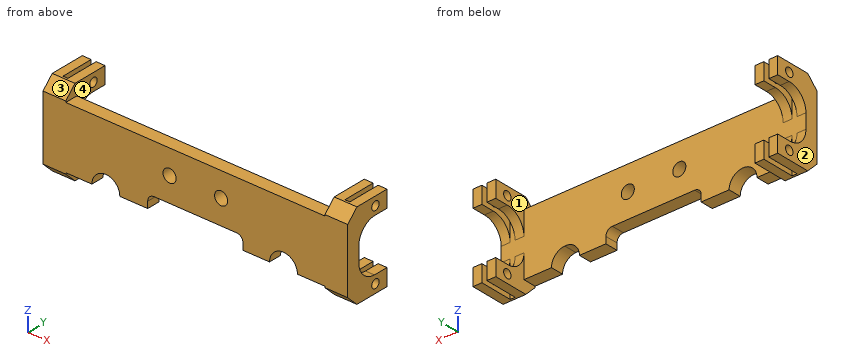
from build123d import *

# Parameters (mm, degrees)
BOSS_EXTRUDE1_DEPTH      = 3
SKETCH2_W                = 14.396583112
SKETCH2_H                = 3
BOSS_EXTRUDE2_DEPTH      = 8.6
SKETCH3_R                = 1
BOSS_EXTRUDE3_DEPTH      = 5.3
SKETCH4_W                = 1.15
SKETCH4_H                = 7.632118098
CUT_EXTRUDE1_DEPTH       = 26.3
CHAMFER1_SIZE            = 2.5
CUT_EXTRUDE2_DEPTH       = 10
CHAMFER1_OF_MIRROR1_SIZE = 2.5
CUT_EXTRUDE5_START       = -10
CUT_EXTRUDE5_DEPTH       = 10
BOSS_EXTRUDE4_DEPTH      = 3
SKETCH7_R                = 1.525
CUT_EXTRUDE6_DEPTH       = 41.163420863


with BuildPart() as part:
    # Sketch1 → Boss-Extrude1 (new body)
    with BuildSketch(Plane(origin=(0, 0, 0), x_dir=(1, 0, 0), z_dir=(0, 1, 0))):
        with BuildLine():
            Line((-26.88337521, 0), (-26.88337521, 14.396583112))
            Line((-26.88337521, 14.396583112), (-24.09337521, 14.396583112))
            ThreePointArc((-24.09337521, 14.396583112), (-20.84337521, 11.146583112), (-17.59337521, 14.396583112))
            Line((-17.59337521, 14.396583112), (0, 14.396583112))
            Line((0, 14.396583112), (0, 0))
            Line((0, 0), (-26.88337521, 0))
        make_face()
    boss_extrude1 = extrude(amount=BOSS_EXTRUDE1_DEPTH)

    # Sketch2 → Boss-Extrude2 (add)
    with BuildSketch(Plane.ZY.offset(26.88337521)):
        with Locations((-7.198291556, 1.5)):
            Rectangle(SKETCH2_W, SKETCH2_H)
    boss_extrude2 = extrude(amount=BOSS_EXTRUDE2_DEPTH)

    # Sketch3 → Boss-Extrude3 (add)
    with BuildSketch(Plane.ZY.offset(35.48337521)):
        with BuildLine():
            Line((1.532781983, 10.632118098), (-1.123291556, 10.632118098))
            Line((-1.123291556, 10.632118098), (-1.123291556, 10.557118098))
            Line((-1.123291556, 10.557118098), (-1.123291556, 7.547815402))
            ThreePointArc((-1.123291556, 7.547815402), (-2.349871735, 4.342215517), (-5.508799885, 3))
            Line((-5.508799885, 3), (-8.887750376, 3))
            ThreePointArc((-8.887750376, 3), (-11.934395079, 4.229921298), (-13.273291556, 7.230272374))
            Line((-13.273291556, 7.230272374), (-13.273291556, 10.557118098))
            Line((-13.273291556, 10.557118098), (-13.273291556, 10.632118098))
            Line((-13.273291556, 10.632118098), (-15.929365096, 10.632118098))
            Line((-15.929365096, 10.632118098), (-17.198291556, 10.632118098))
            Line((-17.198291556, 10.632118098), (-17.198291556, 7.5))
            Line((-17.198291556, 7.5), (-17.198291556, 0))
            Line((-17.198291556, 0), (-14.396583112, 0))
            Line((-14.396583112, 0), (0, 0))
            Line((0, 0), (2.801708444, 0))
            Line((2.801708444, 0), (2.801708444, 7.5))
            Line((2.801708444, 7.5), (2.801708444, 10.632118098))
            Line((2.801708444, 10.632118098), (1.532781983, 10.632118098))
        make_face()
        with Locations((-15.198291556, 7.5)):
            Circle(SKETCH3_R, mode=Mode.SUBTRACT)
        with Locations((0.801708444, 7.5)):
            Circle(SKETCH3_R, mode=Mode.SUBTRACT)
    boss_extrude3 = extrude(amount=-BOSS_EXTRUDE3_DEPTH)

    # Sketch4 → Cut-Extrude1 (cut)
    with BuildSketch(Plane.XY.offset(2.801708444)):
        with Locations((-32.83337521, 6.816059049)):
            Rectangle(SKETCH4_W, SKETCH4_H)
    cut_extrude1 = extrude(amount=-CUT_EXTRUDE1_DEPTH, mode=Mode.SUBTRACT)

    # Chamfer1
    chamfer1_edges = [part.edges().sort_by_distance(p)[0] for p in [
        (-32.83337521, 0, -17.198291556),
        (-32.83337521, 0, 2.801708444),
    ]]
    chamfer(chamfer1_edges, length=CHAMFER1_SIZE)

    # Sketch5 → Cut-Extrude2 (cut)
    with BuildSketch(Plane(origin=(0, 3, 0), x_dir=(1, 0, 0), z_dir=(0, 1, 0))):
        with BuildLine():
            Line((0, 11.381166784), (-9.598972409, 11.381166784))
            ThreePointArc((-9.598972409, 11.381166784), (-10.65963258, 11.820506612), (-11.098972409, 12.881166784))
            Line((-11.098972409, 12.881166784), (-11.098972409, 14.396583112))
            Line((-11.098972409, 14.396583112), (0, 14.396583112))
            Line((0, 14.396583112), (0, 11.381166784))
        make_face()
    cut_extrude2 = extrude(amount=-CUT_EXTRUDE2_DEPTH, mode=Mode.SUBTRACT)

    # Mirror1: Boss-Extrude1, Boss-Extrude2, Boss-Extrude3, Cut-Extrude1, Cut-Extrude2 across plane
    add(boss_extrude1.mirror(Plane(origin=(0, 0, 0), x_dir=(0, 0, 1), z_dir=(1, 0, 0))))
    add(boss_extrude2.mirror(Plane(origin=(0, 0, 0), x_dir=(0, 0, 1), z_dir=(1, 0, 0))))
    add(boss_extrude3.mirror(Plane(origin=(0, 0, 0), x_dir=(0, 0, 1), z_dir=(1, 0, 0))))
    add(cut_extrude1.mirror(Plane(origin=(0, 0, 0), x_dir=(0, 0, 1), z_dir=(1, 0, 0))), mode=Mode.SUBTRACT)
    add(cut_extrude2.mirror(Plane(origin=(0, 0, 0), x_dir=(0, 0, 1), z_dir=(1, 0, 0))), mode=Mode.SUBTRACT)

    # Chamfer1 of Mirror1
    chamfer1_of_mirror1_edges = [part.edges().sort_by_distance(p)[0] for p in [
        (32.83337521, 0, -17.198291556),
        (32.83337521, 0, 2.801708444),
    ]]
    chamfer(chamfer1_of_mirror1_edges, length=CHAMFER1_OF_MIRROR1_SIZE)

    # Sketch6 → Cut-Extrude5 (cut)
    with BuildSketch(Plane(origin=(0, 3, 0), x_dir=(1, 0, 0), z_dir=(0, 1, 0)).offset(CUT_EXTRUDE5_START)):
        with BuildLine():
            ThreePointArc((20.68337521, 11.150523963), (22.877361191, 12.155768528), (23.77337521, 14.396583112))
            ThreePointArc((23.77337521, 14.396583112), (20.52337521, 17.646583112), (17.27337521, 14.396583112))
            Line((17.27337521, 14.396583112), (17.59337521, 14.396583112))
            ThreePointArc((17.59337521, 14.396583112), (18.489389228, 12.155768528), (20.68337521, 11.150523963))
        make_face()
        with BuildLine():
            Line((17.59337521, 14.396583112), (17.27337521, 14.396583112))
            ThreePointArc((17.27337521, 14.396583112), (18.282560626, 12.042597131), (20.68337521, 11.150523963))
            ThreePointArc((20.68337521, 11.150523963), (18.489389228, 12.155768528), (17.59337521, 14.396583112))
        make_face()
    extrude(amount=CUT_EXTRUDE5_DEPTH, mode=Mode.SUBTRACT)

    # Sketch6<3> → Boss-Extrude4 (add, through all)
    with BuildSketch(Plane(origin=(0, 3, 0), x_dir=(1, 0, 0), z_dir=(0, 1, 0))):
        with BuildLine():
            Line((24.09337521, 14.396583112), (23.77337521, 14.396583112))
            ThreePointArc((23.77337521, 14.396583112), (22.877361191, 12.155768528), (20.68337521, 11.150523963))
            ThreePointArc((20.68337521, 11.150523963), (20.763350947, 11.147568474), (20.84337521, 11.146583112))
            ThreePointArc((20.84337521, 11.146583112), (23.141472249, 12.098486073), (24.09337521, 14.396583112))
        make_face()
    extrude(amount=-BOSS_EXTRUDE4_DEPTH)

    # Sketch7 → Cut-Extrude6 (cut, through all)
    with BuildSketch(Plane(origin=(0, 3, 0), x_dir=(1, 0, 0), z_dir=(0, 1, 0))):
        with Locations(Location((-6, 5.690583392, 0), (0, 0, 270))):
            Circle(SKETCH7_R)
        with Locations(Location((6, 5.690583392, 0), (0, 0, 90))):
            Circle(SKETCH7_R)
    extrude(amount=-CUT_EXTRUDE6_DEPTH, mode=Mode.SUBTRACT)


solid = part.part
CAD build for the part. Positions are in the model's coordinates, mm. Face numbers are marked on the shaded views. Coordinates: 2 decimals unless noted, no trailing zeros. Loops run counter-clockwise (first coordinate to the right, second up) from the corner with the lowest first, then second, coordinate; pieces in that order, holes last. Notation, with made-up numbers: (-26, 4) - (-14, 4) arc R27 ccw to (-14, 20) - close; hole circle Ø5 at (-10, 73). An arc over 180 degrees is marked (long way). Write item = value, one per line. Start each with the question number.
Q1. Drill centre lines: L1, parallel to X at y = 4.25, z = -16.5; L2, parallel to Z at x = 34.8, y = 7.5; L3, parallel to Z at x = 6, y = 2.45. Where is each one in solid material? Low to high.
Q2. Cut at C-C, the plane z = -12. List the corners of the cut face in (x, y), then the cut area to 3 significant figures.
Q3. Cut at D-D, the plane x = -25. List the corners of the cut face in (y, z).
Q4. Pull direction X, two halves, no side cores. Call the marked faces 1, 2, 3 and 4: pulls with the +X half, pulls with the -X half, needs draft (parallel to the pull), parting line crosses it, or undercut.
Q5. Cut at A-A, the plane y = 9.5. Give the number of separate pieces and of enclosed holes in the cut face, then the cut area to 3 significant figures.
Q6. Cut at B-B, the plane x = 6. List the corners of the cut face in (y, z), then the cut area to 3 significant figures.
Q7. Flat gauge pins, fed straight in: pin 1 Ø3 at (x, z) = (-4, -3) entering from -Y; pin 2 Ø1.2 at (y, z) = (7.5, 0.8) entering from -X; pin 3 Ø2.5 at (x, y) = (-12.5, 2) entering from -Z. Where does each tip first touch, or does it go through?
Computed:
q1.L1 = -35.48 to -33.41, -32.26 to -30.18, 30.18 to 32.26, 33.41 to 35.48
q1.L2 = -17.2 to -16.2, -14.2 to -13.27, -1.12 to -0.2, 1.8 to 2.8
q1.L3 = -11.38 to -7.22, -4.17 to 0
q2.outline = (-35.48, 0) - (-23.04, 0) - (-23.04, 3) - (-30.18, 3) - (-30.18, 4.29) - (-32.26, 4.29) - (-32.26, 3) - (-33.41, 3) - (-33.41, 4.29) - (-35.48, 4.29) - close; (-18.65, 0) - (-10.81, 0) - (-10.81, 3) - (-18.65, 3) - close; (10.81, 0) - (18.33, 0) - (18.33, 3) - (10.81, 3) - close; (22.72, 0) - (35.48, 0) - (35.48, 4.29) - (33.41, 4.29) - (33.41, 3) - (32.26, 3) - (32.26, 4.29) - (30.18, 4.29) - (30.18, 3) - (22.72, 3) - close
q2.area = 132 mm²
q3.outline = (0, -14.4) - (3, -14.4) - (3, 0) - (0, 0) - close
q4.face_1 = undercut
q4.face_2 = pulls with the -X half
q4.face_3 = needs draft
q4.face_4 = undercut
q5.separate_pieces = 8
q5.enclosed_holes = 0
q5.area = 65.2 mm²
q6.outline = (0, -11.38) - (3, -11.38) - (3, -7.22) - (0, -7.22) - close; (0, -4.17) - (3, -4.17) - (3, 0) - (0, 0) - close
q6.area = 25.0 mm²
q7.pin_1 = 0
q7.pin_2 = through
q7.pin_3 = -14.4
